For this review, take the finished solid that the model builds, in its own axes (mm). A direction names the side the tool comes from. Give positions to 0.01 mm unless a question says otherwise; leave off trailing zeros. Order: outer loops, then holes, each group sorted by start corner. A loop starts at its lowest first (then second) coordinate and runs counter-clockwise, first axis right, second up.
Item 1: The part is to be moulded in two halves that separate along X. For faces 4 (the cylindrical face through (28.584, 6.261, -0.419)), 5 (the cylindrical face through (-69.842, 6.261, 0.698)), 6 (the flat face through (-1, 12, -31.75)), say which applies: released by +X, released by -X, zero draft, split by the parting line, or undercut.
Item 2: For P1, Ø6, axis at y = 9, z = 6, coming from the -X side; P2, Ø15, axis at y = 31.75, z = 0, coming from the +X side; P3, Ø12, axis at x = -49.5, y = 14.5, coming from the -Z side; P4, Ø2, axis at x = 48, y = 7.5, coming from the +Z side, all flat-tipped, find the tip position at first contact; note any pin that passes through.
Item 3: For probe 1 along X at (y, z) = (4.5, 0) (3 decimals); probe 2 along X at (y, z) = (7, 2); probe 3 along Y at (x, z) = (-8, 0), list the stretches that pass through material, from the lowest coordinate up.
Item 4: Consider section D-D (x = 33). Give the boundary of the cut face in (y, z).
Item 5: Machinability: for faces 1 (the flat face through (-22.225, 43, -7)), 2 (the flat face through (1, 0, 0)), 3 (the flat face through (22.225, 43, -7)), which of the approach directions +Z, -Z, +X, -X, +Y, -Y give a long, thin tool a straight path to every point of the face, cutting with its end or side? Answer none if there is none.
Item 6: Consider section C-C (y = 26.5). Give the boundary of the cut face in (x, z) (3 decimals), plus the area to 3 significant figures.
Item 7: Consider section B-B (z = 11). Give the boundary of the cut face in (x, y) (3 decimals).
Item 8: Consider section A-A (x = 1). Give the boundary of the cut face in (y, z), plus the area to 3 significant figures.
```python
from build123d import *

# Parameters (mm, degrees)
SKETCH1_R           = 9.525
BOSS_EXTRUDE2_DEPTH = 12.7
SKETCH2_W           = 44.45
SKETCH2_H           = 63.5
BOSS_EXTRUDE3_DEPTH = 19.05
BOSS_EXTRUDE4_DEPTH = 44.45
SKETCH4_R           = 12.7
CUT_EXTRUDE1_DEPTH  = 44.45


with BuildPart() as part:
    # Sketch1 → Boss-Extrude2 (new body)
    with BuildSketch(Plane(origin=(0, 0, 0), x_dir=(1, 0, 0), z_dir=(0, 1, 0))):
        with BuildLine():
            Line((-38.1, 31.75), (38.1, 31.75))
            ThreePointArc((38.1, 31.75), (69.85, 0), (38.1, -31.75))
            Line((38.1, -31.75), (-38.1, -31.75))
            ThreePointArc((-38.1, -31.75), (-69.85, 0), (-38.1, 31.75))
        make_face()
        with Locations((-38.1, 0)):
            Circle(SKETCH1_R, mode=Mode.SUBTRACT)
        with Locations((38.1, 0)):
            Circle(SKETCH1_R, mode=Mode.SUBTRACT)
    extrude(amount=BOSS_EXTRUDE2_DEPTH)

    # Sketch2 → Boss-Extrude3 (add)
    with BuildSketch(Plane(origin=(0, 12.7, 0), x_dir=(1, 0, 0), z_dir=(0, 1, 0))):
        Rectangle(SKETCH2_W, SKETCH2_H)
    extrude(amount=BOSS_EXTRUDE3_DEPTH)

    # Sketch3 → Boss-Extrude4 (add)
    with BuildSketch(Plane(origin=(22.225, 0, 0), x_dir=(0, 0, -1), z_dir=(1, 0, 0))):
        with BuildLine():
            Line((-31.75, 12.7), (31.75, 12.7))
            Line((31.75, 12.7), (31.75, 31.75))
            ThreePointArc((31.75, 31.75), (0, 63.5), (-31.75, 31.75))
            Line((-31.75, 31.75), (-31.75, 12.7))
        make_face()
    extrude(amount=-BOSS_EXTRUDE4_DEPTH)

    # Sketch4 → Cut-Extrude1 (cut)
    with BuildSketch(Plane(origin=(22.225, 0, 0), x_dir=(0, 0, -1), z_dir=(1, 0, 0))):
        with Locations((0, 31.75)):
            Circle(SKETCH4_R)
    extrude(amount=-CUT_EXTRUDE1_DEPTH, mode=Mode.SUBTRACT)


solid = part.part
```
Resolved:
1. face 4: undercut
1. face 5: released by -X
1. face 6: zero draft
2. P1: stops at x = -69.71
2. P2: passes through
2. P3: stops at z = -31.24
2. P4: stops at z = 30.48
3. probe 1: x = -69.85 to -47.625, -28.575 to 28.575, 47.625 to 69.85
3. probe 2: x = -69.79 to -47.41, -28.79 to 28.79, 47.41 to 69.79
3. probe 3: y = 0 to 19.05, 44.45 to 63.5
4. outline: (0, -31.75) - (12.7, -31.75) - (12.7, -8.04) - (0, -8.04) - close; (0, 8.04) - (12.7, 8.04) - (12.7, 31.75) - (0, 31.75) - close
5. face 1: +Z, -Z, -X, +Y
5. face 2: +Z, -Z, +X, -X, -Y
5. face 3: +Z, -Z, +X, +Y
6. outline: (-22.225, -31.75) - (22.225, -31.75) - (22.225, -11.564) - (-22.225, -11.564) - close; (-22.225, 11.564) - (22.225, 11.564) - (22.225, 31.75) - (-22.225, 31.75) - close
6. area: 1,790 mm2
7. outline: (-67.884, 0) - (67.884, 0) - (67.884, 12.7) - (22.225, 12.7) - (22.225, 25.403) - (-22.225, 25.403) - (-22.225, 12.7) - (-67.884, 12.7) - close; (-22.225, 38.097) - (22.225, 38.097) - (22.225, 61.534) - (-22.225, 61.534) - close
8. outline: (0, -31.75) - (31.75, -31.75) arc R31.75 ccw to (31.75, 31.75) - (0, 31.75) - close; hole circle Ø25.4 at (31.75, 0)
8. area: 3,090 mm2
